Verification items for the finished model (mm, model axes). A direction names the side the tool comes from. Coordinates: 2 decimals unless noted, no trailing zeros. Loops run counter-clockwise (first coordinate to the right, second up) from the corner with the lowest first, then second, coordinate; pieces in that order, holes last. Notation, with made-up numbers: (22, 3.5) -> (27, 3.5) arc R20 ccw to (27, 41.5) -> close; hole circle Ø1 at (53.25, -24.5). An arc over 180 degrees is marked (long way). Use CSV: the item, a comma, the result in double quotes. Start each with the question number.
Autodesk Inventor part; units mm, degrees
ref_plane "Work Plane1" through (29, 0, 0) normal (0, -1, 0) x (1, 0, 0)
ref_plane "YZ Plane" through (0, 0, 0) normal (1, 0, 0) x (0, 1, 0)
ref_plane "XZ Plane" through (0, 0, 0) normal (0, 1, 0) x (-1, 0, 0)
sketch "Sketch1" plane through (0, 0, 0) normal (0, 0, 1) x (1, 0, 0)
  line L0 (-2, 0) -> (30, 0)
  line L1 (30, 0) -> (30, 4)
  line L2 (30, 4) -> (3.125, 4)
  line L3 (3.125, 4) -> (2.3581, 4)
  line L4 (2.3581, 4) -> (0, 4)
  line L5 (0, 4) -> (0, 6.5)
  line L6 (0, 6.5) -> (-8, 6.5)
  line L7 (-8, 6.5) -> (-8, 3.4641)
  line L8 (-8, 3.4641) -> (-4, 3.4641)
  line L9 (-4, 3.4641) -> (-2, 0)
  line L10 (-11.8, 0) -> (41.4, 0)
  line L11 (0, -0.65) -> (0, 8.45)
  line L12 (3.125, 4) -> (0, 4) construction
  dimension "d1" = 26.875
  dimension "d2" = 0.7669
  dimension "d3" = 8
  dimension "d4" = 4
  dimension "d5" = 60
  dimension "d6" = 8
  dimension "d7" = 8
  dimension "d8" = 6.9282
  dimension "d9" = 13
  dimension "d26" = 30
revolve "Body" add sketch "Sketch1" angle 360 about axis through (-2, 0, 0) along (1, 0, 0)
sketch "Sketch2" plane through (-8, 0, 0) normal (-1, 0, 0) x (0, 0, 1)
  circle A0 centre (0, 0) radius 3.4641
  line L0 (0, -7.8) -> (0, 10.4)
  line L1 (-7.8, 0) -> (10.4, 0)
  line L2 (3.4641, 0) -> (1.7321, -3)
  line L3 (1.7321, -3) -> (-1.7321, -3)
  line L4 (-1.7321, -3) -> (-3.4641, 0)
  line L5 (-3.4641, 0) -> (-1.7321, 3)
  line L6 (-1.7321, 3) -> (1.7321, 3)
  line L7 (1.7321, 3) -> (3.4641, 0)
extrude "Slot" add sketch "Sketch2" against normal up to next contours L7 A0 | A0 L2 | L6 L0 A0 | A0 L0 L3 | L0 L6 A0 | A0 L3 L0 | L4 A0 | A0 L5
fillet "Fillet1" radius 0.8 1 edges at (-8, -6.5, 0)
thread "Thread"
chamfer "Chamfer1" distance 0.7668 distance2 0.7668 1 edges at (30, -4, 0) measured on face at (30, -0.4013, -0.6579)
ref_plane "Work Plane1" through (29, 0, 0) normal (0, -1, 0) x (1, 0, 0)
equation "\"d1\" = GEL"
equation "\"d3\" = KOH"
equation "\"d4\" = INTI"
equation "\"d6\" = GD"
equation "\"d7\" = BDM"
equation "\"d8\" = 1.1547 * SW"
equation "\"d9\" = KOD"
equation "\"d26\" = NLG"
equation "\"d17\" = RR"
equation "\"d13\" = GEL"
equation "\"d15\" = -0.5 * SPD + 0.5 * GD"
equation "\"d16\" = GUL"
equation "\"GD\" = 8"
equation "\"NLG\" = 30"
equation "\"GEL\" = 26.875"
equation "\"KOD\" = 13"
equation "\"KOH\" = 8"
equation "\"INTI\" = 4"
equation "\"GAL\" = 0.61345 * PTC"
equation "\"GUL\" = 0.61345 * PTC"
equation "\"BDM\" = NND"
equation "\"SW\" = 6"
equation "\"RR\" = 0.8"
equation "\"SPD\" = NND - 1.2269 * PTC"
equation "\"TOA\" = 30deg"
equation "\"GD1\" = THREADDIA - 1.2269 * PTC"
equation "\"THREADDIA\" = 8"
equation "\"FAWI\" = 45deg"
equation "\"PTC\" = 1.25"
equation "\"NND\" = 8"
equation "\"E0\" = 1.155 * SW"
properties part number "100001" material "Steel, Mild"
1. Cross-section at B-B, the plane x = 9. Record the boundary of the cut face in (y, z).
2. Scan lines: line 1 (X direction, y = 1, z = -4.5); line 2 (Y direction, x = -5, z = 3.25); line 3 (Y direction, x = 7, z = -2). Record each from-to range of solid material in increasing order.
3. Set-up check for faces 4 (the flat face through (0, 3, 3)), 5 (the flat face through (-5.9, -1.5, -2.6)), 6 (the flat face through (-8, -2.5, 2.5)): record each of +Z, -Z, +X, -X, +Y, -Y from which the full face is reachable in a straight line by a thin tool's end or side.
4. Release check for a two-part mould opening along Y. For faces 1 (the flat face through (-5.9, -1.5, 2.6)), 2 (the cylindrical face through (14.412, -0.867, 3.905)), 3 (the flat face through (30, 0, 0)) record: released by +Y, released by -Y, zero draft, split by the parting line, or undercut.
5. Cross-section at A-A, the plane x = -5.5. Record the boundary of the cut face in (y, z), plus the area to 3 significant figures.
6. Depth check by flat-ended pin: pin 1 (1.5 mm diameter, centred on y = 0, z = 2.5, fed in from -X); pin 2 (1.5 mm diameter, centred on x = 3, z = 4, fed in from -Y); pin 3 (6 mm diameter, centred on x = -2, z = 3.5, fed in from +Y); pin 4 (4 mm diameter, centred on x = -5, z = -0.5, fed in from -Y). Enter the tip coordinate at first touch or a pass-through.
Solution:
1,outline,"circle Ø8 at (0, 0)"
2,line 1,"x = -8 to 0"
2,line 2,"y = -5.63 to -0.37, 0.37 to 5.63"
2,line 3,"y = -3.46 to 3.46"
3,face 4,"+X"
3,face 5,"-X"
3,face 6,"+Z, -Z, -X, +Y, -Y"
4,face 1,"undercut"
4,face 2,"split by the parting line"
4,face 3,"zero draft"
5,outline,"circle Ø13 at (0, 0); hole (-3, -1.73) -> (0, -3.46) -> (3, -1.73) -> (3, 1.73) -> (0, 3.46) -> (-3, 1.73) -> close"
5,area,"102 mm2"
6,pin 1,"stops at x = -3.88"
6,pin 2,"stops at y = -2.33"
6,pin 3,"stops at y = 6.48"
6,pin 4,"stops at y = -6.5"
